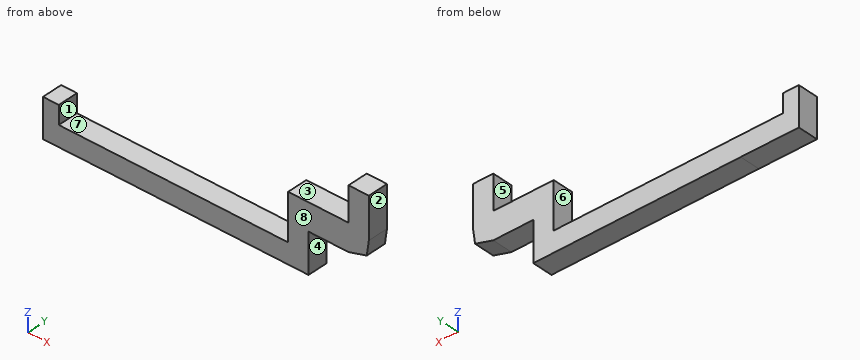
from build123d import *

# Parameters (mm, degrees)
F0_W     = 3.8658287376
F0_H     = 4.4971403014
F1_DEPTH = 5


with BuildPart() as f1:
    # F0 (on Front) → F1 (new body)
    with BuildSketch(Plane.XZ):
        Polygon((-27.5305788964, -12.3905977234), (-13.2927056402, -12.3482672498), (37.4694211036, -12.3482672498), (37.4694211036, -2.6401227806), (47.2564931819, -2.6401227806), (51.7159264395, -1.3378107687), (52.2289585182, 2.292877296), (52.2289585182, 12.3167335987), (47.2564931819, 12.3167335987), (47.2564931819, 3.9355711732), (32.4694211036, 3.9355711732), (32.4694211036, -7.3905977234), (-10.1355845109, -7.3905977234), (-23.6647501588, -7.3905977234), (-27.5305788964, -7.3905977234), align=None)
        with Locations((-25.5976645276, -5.1420275727)):
            Rectangle(F0_W, F0_H)
    extrude(amount=F1_DEPTH)


solid = f1.part
Design review of the part built by this model. Coordinates are the model's own, in mm. Face numbers are marked on the shaded views. A direction names the side the tool comes from. Give positions to 0.01 mm unless a question says otherwise; leave off trailing zeros. Loops run counter-clockwise (first coordinate to the right, second up) from the corner with the lowest first, then second, coordinate; pieces in that order, holes last. Notation, with made-up numbers: M 16.5,80.5 L 54.5,80.5 A30 ccw 54.5,108.5 Z; hole C 72.5,30 d9. An arc over 180 degrees is marked long. Write item = value, one per line.
Q1. Insertion check: pin 1 (1.5 mm diameter, centred on y = -3, z = -6.5, fed in from +X); pin 2 (2.5 mm diameter, centred on x = 43, y = -2.5, fed in from +Z); pin 3 (4 mm diameter, centred on x = 31.5, z = 7, fed in from -Y); pin 4 (1.5 mm diameter, centred on x = -6, y = -3, fed in from +Z). Each pin has a flat end and moves straight along its axis. Give the tip position at first contact, or say it passes through.
Output values:
pin_1 = 37.47
pin_2 = 3.94
pin_3 = through
pin_4 = -7.39
Q2. Draft analysis for pull direction X (two halves, no side actions). For the marked faces 5, 6, 7 and 8, state which applies: +X half, -X half, draft (parallel to the pull), parting line (faces both ways), or undercut.
Output values:
face_5 = -X half
face_6 = undercut
face_7 = undercut
face_8 = draft
Q3. We need section D-D (z = 8). Give the boundary of the cut face in (x, y), plus the area to 3 significant figures.
Output values:
outline = M 47.26,-5 L 52.23,-5 L 52.23,0 L 47.26,0 Z
area = 24.9 mm^2
Q4. We need section B-B (y = -3.25). Give the boundary of the cut face in (x, z), plus the area to 3 significant figures.
Output values:
outline = M -27.53,-12.39 L -13.29,-12.35 L 37.47,-12.35 L 37.47,-2.64 L 47.26,-2.64 L 51.72,-1.34 L 52.23,2.29 L 52.23,12.32 L 47.26,12.32 L 47.26,3.94 L 32.47,3.94 L 32.47,-7.39 L -23.66,-7.39 L -23.66,-2.89 L -27.53,-2.89 Z
area = 531 mm^2
Q5. We need section C-C (x = 36). Give the boundary of the cut face in (y, z).
Output values:
outline = M -5,-12.35 L 0,-12.35 L 0,3.94 L -5,3.94 Z
Q6. We need section A-A (z = -5.25). Give the boundary of the cut face in (x, y).
Output values:
outline = M -27.53,-5 L -23.66,-5 L -23.66,0 L -27.53,0 Z; M 32.47,-5 L 37.47,-5 L 37.47,0 L 32.47,0 Z
Q7. For the marked faces 1, 2, 3 and 4, list the 3-axis set-ups (+Z, -Z, +X, -X, +Y, -Y) from which the entire face can be reached by the end or side of a thin tool; tool diameter is ignored.
Output values:
face_1 = +Z, +Y, -Y
face_2 = +Z, -Z, +X, +Y, -Y
face_3 = +Z, -X, +Y, -Y
face_4 = -Z, +X, +Y, -Y
Q8. To check wall thickness, follow line 1 (X direction, y = -2.2, z = -5); line 2 (Z direction, x = 29.5, y = -1.1); line 3 (X direction, y = -2.45, z = 4). State the ranges of each line that lie inside material, in increasing order. Write a range as [from, to].
Output values:
line_1 = [-27.53, -23.66], [32.47, 37.47]
line_2 = [-12.35, -7.39]
line_3 = [47.26, 52.23]
